Could you check a few things on this drawing? It's one solid part, dimensions in mm from its lowest x, y, z. Coordinates: 2 decimals unless noted, no trailing zeros. Loops run counter-clockwise (first coordinate to the right, second up) from the corner with the lowest first, then second, coordinate; pieces in that order, holes last.
1) Imagine slicing it at B-B on y = 24.5. Please give me the cut outline in (x, z), plus the area to 3 significant figures.
2) If I drill on line 1 along Y through (x, z) = (24.5, 4); line 2 along Y through (x, z) = (16, 5) (1 decimal); line 3 along Z through (x, y) = (42, 40), over which ranges is the centre line in solid material (lowest first)?
3) Thinking about a two-plate mould opening in X: for the marked faces 1, 2 and 3, which applies, released by +X, released by -X, zero draft, split by the parting line, or undercut?
4) Will these pins go through, and if not, where does the flat tip stop? P1, Ø3, axis at x = 24.5, y = 39.2, coming from the +Z side; P2, Ø6, axis at x = 32, y = 22.5, coming from the -Z side; P3, Ø1.5, axis at y = 17, z = 5.5, coming from the +X side; P4, Ø3, axis at x = 8, y = 5, coming from the +Z side.
5) Imagine slicing it at D-D on z = 4.5. Please give me the cut outline in (x, y).
6) Imagine slicing it at A-A on x = 24.5. Please give me the cut outline in (y, z).
7) Imagine slicing it at C-C on x = 33.5. Please give me the cut outline in (y, z), plus the area to 3 significant figures.
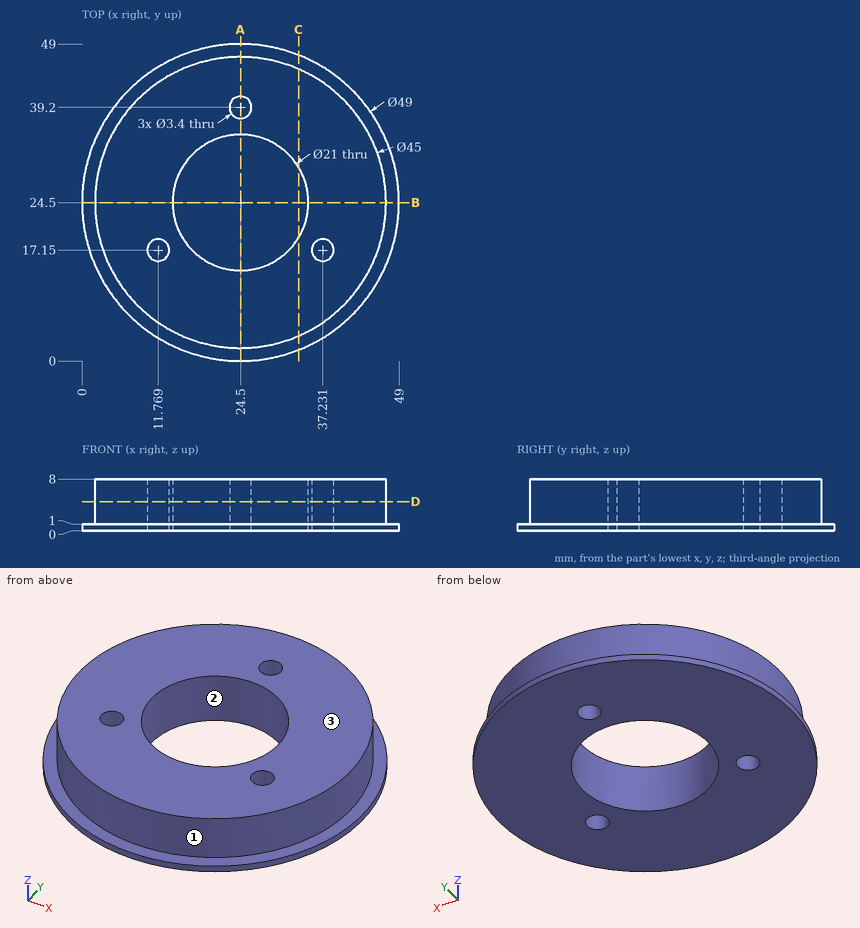
Filled in:
1. outline: (0, 0) - (14, 0) - (14, 8) - (2, 8) - (2, 1) - (0, 1) - close; (35, 0) - (49, 0) - (49, 1) - (47, 1) - (47, 8) - (35, 8) - close
1. area: 196 mm2
2. line 1: y = 2 to 14, 35 to 37.5, 40.9 to 47
2. line 2: y = 3.7 to 18.3, 30.7 to 45.3
2. line 3: z = 0 to 1
3. face 1: split by the parting line
3. face 2: undercut
3. face 3: zero draft
4. P1: passes through
4. P2: stops at z = 0
4. P3: stops at x = 45.96
4. P4: stops at z = 1
5. outline: circle Ø45 at (24.5, 24.5); hole circle Ø3.4 at (11.77, 17.15); hole circle Ø21 at (24.5, 24.5); hole circle Ø3.4 at (24.5, 39.2); hole circle Ø3.4 at (37.23, 17.15)
6. outline: (0, 0) - (14, 0) - (14, 8) - (2, 8) - (2, 1) - (0, 1) - close; (35, 0) - (37.5, 0) - (37.5, 8) - (35, 8) - close; (40.9, 0) - (49, 0) - (49, 1) - (47, 1) - (47, 8) - (40.9, 8) - close
7. outline: (1.71, 0) - (19.09, 0) - (19.09, 8) - (3.88, 8) - (3.88, 1) - (1.71, 1) - close; (29.91, 0) - (47.29, 0) - (47.29, 1) - (45.12, 1) - (45.12, 8) - (29.91, 8) - close
7. area: 248 mm2
